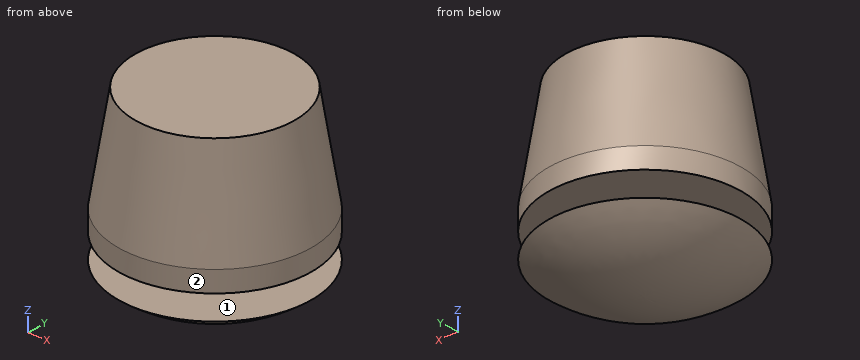
```python
from build123d import *


with BuildPart() as f1:
    # F0 (on Right) → F1 (revolve)
    with BuildSketch(Plane.YZ):
        with BuildLine():
            ThreePointArc((-11.699607, 4.015982), (-6.184838, 1.031946), (0, 0))
            Line((0, 0), (0, 4.7625))
            Line((0, 4.7625), (0, 9.525))
            Line((0, 9.525), (0, 19.05))
            Line((0, 19.05), (0, 22.225))
            Line((0, 22.225), (-9.659656, 22.225))
            Line((-9.659656, 22.225), (-11.699607, 9.525))
            Line((-11.699607, 9.525), (-11.699607, 6.984011))
            Line((-11.699607, 6.984011), (-4.127539, 6.984011))
            Line((-4.127539, 6.984011), (-4.127539, 6.81355))
            Line((-4.127539, 6.81355), (-3.568739, 6.81355))
            Line((-3.568739, 6.81355), (-3.568739, 6.48335))
            Line((-3.568739, 6.48335), (-4.127539, 6.48335))
            Line((-4.127539, 6.48335), (-4.127539, 6.15315))
            Line((-4.127539, 6.15315), (-3.568739, 6.15315))
            Line((-3.568739, 6.15315), (-3.568739, 5.82295))
            Line((-3.568739, 5.82295), (-4.127539, 5.82295))
            Line((-4.127539, 5.82295), (-4.127539, 5.49275))
            Line((-4.127539, 5.49275), (-3.568739, 5.49275))
            Line((-3.568739, 5.49275), (-3.568739, 5.16255))
            Line((-3.568739, 5.16255), (-4.127539, 5.16255))
            Line((-4.127539, 5.16255), (-4.127539, 4.8387))
            Line((-4.127539, 4.8387), (-3.568739, 4.8387))
            Line((-3.568739, 4.8387), (-3.568739, 4.5085))
            Line((-3.568739, 4.5085), (-4.121154, 4.5085))
            Line((-4.121154, 4.5085), (-4.121154, 4.1783))
            Line((-4.121154, 4.1783), (-3.568739, 4.1783))
            Line((-3.568739, 4.1783), (-3.568739, 4.015982))
            Line((-3.568739, 4.015982), (-11.699607, 4.015982))
        make_face()
    revolve(axis=Axis((0, 0, 11.1125), (0, 0, -1)))


solid = f1.part
```
For this review, take the finished solid that the model builds, in its own axes (mm). Face numbers are marked on the shaded views. A direction names the side the tool comes from. Round coordinates to 2 decimals unless told otherwise and drop trailing zeros. Write each loop counter-clockwise with the first axis right and the second up, starting at its lowest first coordinate (ties: lowest second). Pieces come first, ordered by that corner, then holes. Notation, with made-up numbers: (58, 7) -> (85, 7) arc R16 ccw to (85, 19) -> close; hole circle Ø1 at (-12, 26). An arc over 180 degrees is marked (long way). One line per question, with ' | ' between items. Start each with the question number.
(1) Add section B-B, the plane z = 13.5. Write out the cut boundary in (x, y), plus the area to 3 significant figures.
(2) For line 1 along Z through (x, y) = (3.5, 1) (1 decimal); line 2 along Z through (x, y) = (6.5, -1.25) (3 decimals); line 3 along Z through (x, y) = (-1, 5.25) (3 decimals), list the stretches that pass through material, from the lowest coordinate up. Write a range as from..to.
(3) Tool access review of the marked faces 1 and 2: name each direction out of +Z, -Z, +X, -X, +Y, -Y from which nothing blocks a thin tool from reaching the whole face with its end or side.
(4) Insertion check: P1, Ø5, axis at y = 9, z = 14.5, coming from the -X side; P2, Ø1, axis at x = -4.5, z = 8.5, coming from the -Y side; P3, Ø1.5, axis at x = 4, z = 5, coming from the +Y side. Each pin has a flat end and moves straight along its axis. Give the tip position at first contact, or say it passes through.
(5) Add section A-A, the plane z = 17.5. Write out the cut boundary in (x, y).
Answer list:
1) outline: circle Ø22.12 at (0, 0) | area: 384 mm²
2) line 1: 0.4..4, 4.2..4.5, 4.8..5.2, 5.5..5.8, 6.2..6.5, 6.8..22.2 | line 2: 1.187..4.016, 6.984..22.225 | line 3: 0.765..4.016, 6.984..22.225
3) face 1: none | face 2: +Z, -Z
4) P1: x = -8.82 | P2: y = -10.99 | P3: y = 2.54
5) outline: circle Ø20.84 at (0, 0)
